Geometry: final body of the model. Coordinates: model frame, mm. A direction names the side the tool comes from. Give positions to 0.01 mm unless a question says otherwise; leave off trailing zeros. Write each loop counter-clockwise with the first axis right and the second up, starting at its lowest first coordinate (ties: lowest second). Pieces come first, ordered by that corner, then holes. Notation, with made-up numbers: (1, 19.5) -> (19, 19.5) arc R6 cw to (19, 23.5) -> close; hole circle Ø4 at (-12, 25). An arc over 180 degrees is marked (long way). Use CSV: the item, a comma, the result in double quotes. Start each with the question number.
1) Contact query for flat-ended pins moving along their axis: P1, Ø8.5, axis at x = 14.5, y = 29.5, coming from the +Z side; P2, Ø5, axis at y = 35, z = 62.5, coming from the +X side; P3, Ø12, axis at x = 11, z = 88, coming from the +Y side; P4, Ø14.5, axis at y = 23.32, z = 19, coming from the -X side. Output: stop coordinate, or through.
2) Section A-A (z = 19). Output: boundary loops of the cut face in (x, y), plus the area to 3 significant figures.
3) Draft query along Z for faces 5 (the face through (18.116, 8.288, 2.028)), 6 (the face through (-35.884, 17.779, 8.354)), 7 (the face through (-44.771, 23, 33)). Return one class per face: pulls with the +Z half, pulls with the -Z half, needs draft (parallel to the pull), parting line crosses it, or undercut.
4) Set-up query: faces 1 (the face through (-12.02, 8.67, 88.8)), 2 (the face through (9.255, 23, 33)), 3 (the face through (-34, 24, 65)), 4 (the face through (17, 24, 65)). Return all of +Z, -Z, +X, -X, +Y, -Y with unobstructed straight access to the full face (end or side cutting, diameter ignored); none if empty.
5) Section B-B (z = 34). Output: boundary loops of the cut face in (x, y), plus the area to 3 significant figures.
6) Section C-C (x = -38). Output: boundary loops of the cut face in (y, z), plus the area to 3 significant figures.
7) Material intervals for line 1 (X direction, y = 37, z = 13.5); line 2 (Y direction, x = -34, z = 20.5); line 3 (Z direction, x = 23, y = 14), sorted ascending. Write a range as [from, to].
8) Section D-D (y = 14). Count the separate pieces of the cut face and the enclosed holes in it, plus the area to 3 significant figures.
```python
from build123d import *

# Parameters (mm, degrees)
SZKIC1_W                    = 72
SZKIC1_H                    = 34
DODANIE_WYCI_GNI_CIE1_DEPTH = 65
SZKIC3_R                    = 15
DODANIE_WYCI_GNI_CIE2_DEPTH = 40
SZKIC4_W                    = 36
SZKIC4_H                    = 34
WYTNIJ_WYCI_GNI_CIE1_DEPTH  = 45.5
SZKIC6_R                    = 12
WYTNIJ_WYCI_GNI_CIE2_DEPTH  = 73
ZAOKR_GLENIE1_R             = 10
ZAOKR_GLENIE2_R             = 10
ZAOKR_GLENIE3_R             = 10
CHAMFER4_SIZE               = 4
CHAMFER5_SIZE               = 4
CHAMFER6_SIZE               = 2


with BuildPart() as part:
    # Szkic1 → Dodanie-wyciągnięcie1 (new body)
    with BuildSketch(Plane.XY):
        with Locations((-8.770877944, 23.315845824)):
            Rectangle(SZKIC1_W, SZKIC1_H)
    extrude(amount=DODANIE_WYCI_GNI_CIE1_DEPTH)

    # Szkic3 → Dodanie-wyciągnięcie2 (add)
    with BuildSketch(Plane.XY.offset(65)):
        with Locations((-8.770877944, 23.315845824)):
            Circle(SZKIC3_R)
    extrude(amount=DODANIE_WYCI_GNI_CIE2_DEPTH)

    # Szkic4 → Wytnij-wyciągnięcie1 (cut)
    with BuildSketch(Plane(origin=(0, 0, 0), x_dir=(-1, 0, 0), z_dir=(0, 0, -1))):
        with Locations((8.744538928, 23.315845824)):
            Rectangle(SZKIC4_W, SZKIC4_H)
    extrude(amount=-WYTNIJ_WYCI_GNI_CIE1_DEPTH, mode=Mode.SUBTRACT)

    # Szkic6 → Wytnij-wyciągnięcie2 (cut)
    with BuildSketch(Plane.ZY.offset(44.770877944)):
        with Locations(Location((19, 23.315845824, 0), (0, 0, 270))):
            Circle(SZKIC6_R)
    extrude(amount=-WYTNIJ_WYCI_GNI_CIE2_DEPTH, mode=Mode.SUBTRACT)

    # Zaokrąglenie1
    # the kernel refuses this fillet: 10 mm, written as the material it adds along each edge
    with BuildSketch(Plane(origin=(-8.770877944, 23.315845824, 65), x_dir=(1, 0, 0), z_dir=(0, -1, 0))) as zaokr_glenie1_piece_1_section:
        with BuildLine():
            CenterArc((15 + ZAOKR_GLENIE1_R, ZAOKR_GLENIE1_R), ZAOKR_GLENIE1_R, 180, 90)
            Line((15, ZAOKR_GLENIE1_R), (15, 0))
            Line((15, 0), (15 + ZAOKR_GLENIE1_R, 0))
        make_face()
    zaokr_glenie1_piece_1 = revolve(axis=Axis((-8.770877944, 23.315845824, 65), (0, 0, 1)), mode=Mode.PRIVATE)
    zaokr_glenie1_piece_1 = split(zaokr_glenie1_piece_1, bisect_by=Plane(origin=(-26.605426122, 40.315845824, 67.834548177), z_dir=(0, -1, 0)), keep=Keep.TOP, mode=Mode.PRIVATE)
    zaokr_glenie1_piece_1 = split(zaokr_glenie1_piece_1, bisect_by=Plane(origin=(-26.605426122, 6.315845824, 67.834548177), z_dir=(0, 1, 0)), keep=Keep.TOP, mode=Mode.PRIVATE)
    add(zaokr_glenie1_piece_1)

    # Zaokrąglenie2
    zaokr_glenie2_edges = [part.edges().sort_by_distance(p)[0] for p in [
        (-44.770877944, 23.315845824, 65),
    ]]
    fillet(zaokr_glenie2_edges, radius=ZAOKR_GLENIE2_R)

    # Zaokrąglenie3
    zaokr_glenie3_edges = [part.edges().sort_by_distance(p)[0] for p in [
        (27.229122056, 23.315845824, 65),
    ]]
    fillet(zaokr_glenie3_edges, radius=ZAOKR_GLENIE3_R)

    # Chamfer4
    chamfer4_edges = [part.edges().sort_by_distance(p)[0] for p in [
        (18.242291564, 40.315845824, 0),
    ]]
    chamfer(chamfer4_edges, length=CHAMFER4_SIZE)

    # Chamfer5
    chamfer5_edges = [part.edges().sort_by_distance(p)[0] for p in [
        (-35.757708436, 40.315845824, 0),
        (18.242291564, 6.315845824, 0),
        (-35.757708436, 6.315845824, 0),
    ]]
    chamfer(chamfer5_edges, length=CHAMFER5_SIZE)

    # Chamfer6
    chamfer6_edges = [part.edges().sort_by_distance(p)[0] for p in [
        (-23.770877944, 23.315845824, 105),
    ]]
    chamfer(chamfer6_edges, length=CHAMFER6_SIZE)


solid = part.part
```
Answers follow:
1,P1,"stops at z = 66.44"
1,P2,"stops at x = 25.89"
1,P3,"stops at y = 29.26"
1,P4,"passes through"
2,outline,"(-44.77, 6.32) -> (-26.74, 6.32) -> (-26.74, 11.32) -> (-44.77, 11.32) -> close; (-44.77, 35.32) -> (-26.74, 35.32) -> (-26.74, 40.32) -> (-44.77, 40.32) -> close; (9.26, 6.32) -> (27.23, 6.32) -> (27.23, 11.32) -> (9.26, 11.32) -> close; (9.26, 35.32) -> (27.23, 35.32) -> (27.23, 40.32) -> (9.26, 40.32) -> close"
2,area,"360 mm^2"
3,face 5,"pulls with the -Z half"
3,face 6,"undercut"
3,face 7,"needs draft"
4,face 1,"+Z"
4,face 2,"-Z, +Y, -Y"
4,face 3,"+Z, -X"
4,face 4,"+Z, +X"
5,outline,"(-44.77, 6.32) -> (-26.74, 6.32) -> (-26.74, 40.32) -> (-44.77, 40.32) -> close; (9.26, 6.32) -> (27.23, 6.32) -> (27.23, 40.32) -> (9.26, 40.32) -> close"
5,area,"1,220 mm^2"
6,outline,"(6.32, 4) -> (10.32, 0) -> (36.32, 0) -> (40.32, 4) -> (40.32, 64.46) -> (6.32, 64.46) -> close; hole circle Ø24 at (23.32, 19)"
6,area,"1,720 mm^2"
7,line 1,"x = [-44.77, -26.74], [9.26, 27.23]"
7,line 2,"y = [6.32, 11.41], [35.22, 40.32]"
7,line 3,"z = [0, 11.44], [26.56, 63.17]"
8,separate pieces,"3"
8,enclosed holes,"0"
8,area,"3,440 mm^2"
